Can you work these out from the model? Positions are in its coordinate system, mm. Give positions to 0.01 mm unless a question says otherwise; leave off trailing zeros. Order: outer loops, then holes, each group sorted by start corner. A loop starts at its lowest first (then second) coordinate and runs counter-clockwise, first axis right, second up. Notation, with made-up numbers: (-24.75, -8) - (10.25, -8) arc R15 ccw to (10.25, 18) - close; hole circle Ø6 at (64, 51.5). An arc over 180 degrees is marked (long way). Return JSON: item names as keys, results as strings.
```python
from build123d import *

# Parameters (mm, degrees)
F0_W     = 114.3
F0_H     = 257.175
F1_DEPTH = 22.225
F2_W     = 4.7625
F2_H     = 38.1
F3_DEPTH = 257.176
F4_R     = 4.7625
F5_DEPTH = 50.8


with BuildPart() as f1:
    # F0 (on Right) → F1 (new body)
    with BuildSketch(Plane.YZ):
        Rectangle(F0_W, F0_H)
    extrude(amount=F1_DEPTH)

    # F2 (on face) → F3 (cut, through all)
    with BuildSketch(Plane.XY.offset(128.5875)):
        with Locations((2.38125, 0)):
            Rectangle(F2_W, F2_H)
    extrude(amount=-F3_DEPTH, mode=Mode.SUBTRACT)

    # F4 (on face) → F5 (cut)
    with BuildSketch(Plane.XY.offset(128.5875)):
        with Locations((11.1125, -38.1)):
            Circle(F4_R)
        with Locations((11.1125, 38.1)):
            Circle(F4_R)
    extrude(amount=-F5_DEPTH, mode=Mode.SUBTRACT)


solid = f1.part
```
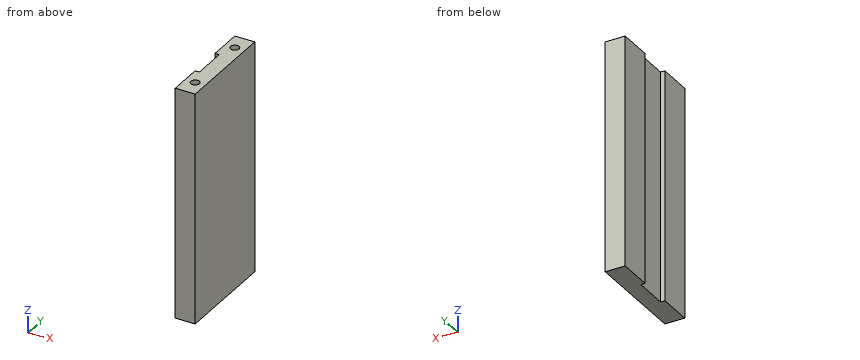
1. For pin 1 Ø5 at (x, y) = (9, -38.5) entering from +Z; pin 2 Ø19 at (y, z) = (-2, -28) entering from -X, each with a flat end and sliding along its axis, tell me the tip position at first contact or that it passes through.
Checks:
{"pin 1": "z = 77.79", "pin 2": "x = 4.76"}
2. Suppose I cut it at C-C (x = 11). List the corners of the cut face in (y, z) for me, plus the area to 3 significant figures.
Checks:
{"outline": "(-57.15, -128.59) - (57.15, -128.59) - (57.15, 128.59) - (42.86, 128.59) - (42.86, 77.79) - (33.34, 77.79) - (33.34, 128.59) - (-33.34, 128.59) - (-33.34, 77.79) - (-42.86, 77.79) - (-42.86, 128.59) - (-57.15, 128.59) - close", "area": "28,400 mm^2"}
3. If I drill on L1, parallel to X at y = 38, z = 107 (3 decimals); L2, parallel to Y at x = 1.25, z = 107; L3, parallel to X at y = 11.5, z = -27 (1 decimal), over which ranges is the centre line in solid material (lowest first)? Write a range as [from, to].
Checks:
{"L1": "[0, 6.351], [15.874, 22.225]", "L2": "[-57.15, -19.05], [19.05, 57.15]", "L3": "[4.8, 22.2]"}
4. Suppose I cut it at D-D (y = -8). List the corners of the cut face in (x, z) for me (1 decimal), plus the area to 3 significant figures.
Checks:
{"outline": "(4.8, -128.6) - (22.2, -128.6) - (22.2, 128.6) - (4.8, 128.6) - close", "area": "4,490 mm^2"}
